The drawing under review shows one solid part. Ordinate dimensions are in mm from its lowest x, y, z. A direction names the side the tool comes from. Give positions to 0.01 mm unless a question says otherwise; leave off trailing zeros. Order: outer loops, then holes, each group sorted by start corner. A loop starts at its lowest first (then second) coordinate and runs counter-clockwise, first axis right, second up. Notation, with made-up numbers: (5, 75) - (50, 75) arc R36 ccw to (50, 114) - close; hole circle Ø9 at (59.25, 59.25). An arc over 180 degrees is marked (long way). Write item = value, one per line. Start each with the question number.
1. For P1, Ø4, axis at y = 31, z = 3.5, coming from the -X side; P2, Ø3, axis at y = 15, z = 4, coming from the -X side; P3, Ø5.5, axis at x = 4.5, z = 9, coming from the +Y side, all flat-tipped, find the tip position at first contact; note any pin that passes through.
2. We need section D-D, the plane x = 20. Give the boundary of the cut face in (y, z).
3. We need section A-A, the plane x = 6.5. Give the boundary of the cut face in (y, z).
4. We need section C-C, the plane y = 19.5. Give the boundary of the cut face in (x, z).
5. We need section B-B, the plane z = 6. State how many separate pieces and enclosed holes the cut face has, and give its area (3 significant figures).
6. Mouldability with a two-part tool opening along X and no side actions: class the marked faces 4, 5 and 6 as pulls with the +X half, pulls with the -X half, needs draft (parallel to the pull), parting line crosses it, or undercut.
7. Wall thickness on probe 1 along X at (y, z) = (23, 5); probe 2 along X at (y, z) = (30, 10); probe 3 along Z at (x, y) = (33.5, 2.75): over which ranges is each line inside the solid? List them lowest first.
8. Machinability: for the marked faces 1, 2 and 3, which of the approach directions +Z, -Z, +X, -X, +Y, -Y give a long, thin tool a straight path to every point of the face, cutting with its end or side? Answer none if there is none.
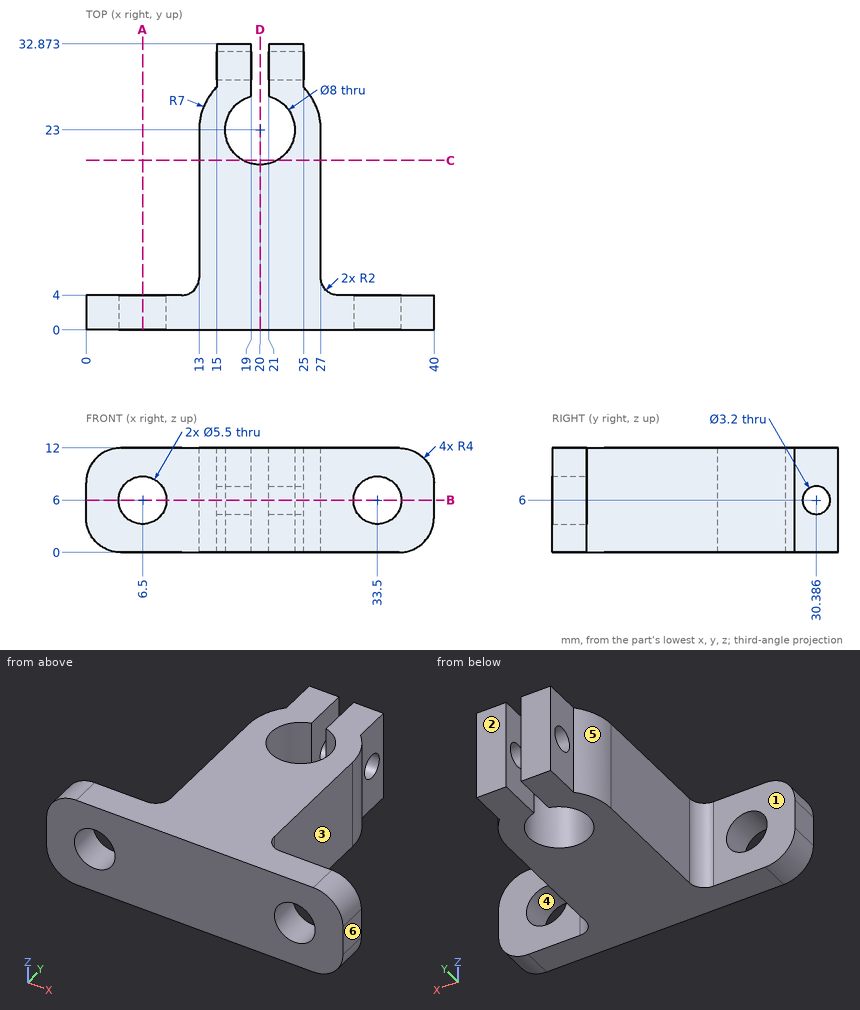
Model answer:
q1.P1 = 15
q1.P2 = 13
q1.P3 = 4
q2.outline = (0, 0) - (19, 0) - (19, 12) - (0, 12) - close
q3.outline = (0, 0) - (4, 0) - (4, 3.25) - (0, 3.25) - close; (0, 8.75) - (4, 8.75) - (4, 12) - (0, 12) - close
q4.outline = (13, 0) - (18.06, 0) - (18.06, 12) - (13, 12) - close; (21.94, 0) - (27, 0) - (27, 12) - (21.94, 12) - close
q5.separate_pieces = 5
q5.enclosed_holes = 0
q5.area = 408 mm2
q6.face_4 = undercut
q6.face_5 = pulls with the -X half
q6.face_6 = pulls with the +X half
q7.probe_1 = 13 to 16, 24 to 27
q7.probe_2 = 15 to 19, 21 to 25
q7.probe_3 = 0 to 3.25, 8.75 to 12
q8.face_1 = +Z, -Z, -X, +Y
q8.face_2 = +Z, -Z, +X, -X, +Y
q8.face_3 = +Z, -Z, +X, +Y
